from build123d import *

# Parameters (mm, degrees)
SKETCH1_R           = 6.35
SKETCH1_R_2         = 3.5814
EXTRUDE1_DEPTH      = 3.175
EXTRUDE1_DEPTH_BACK = 3.175
SKETCH4_W           = 1.1938
SKETCH4_H           = 7.9248
CHAMFER1_SIZE       = 0.254


with BuildPart() as part:
    # Sketch1 → Extrude1 (new, two sides)
    with BuildSketch(Plane(origin=(0, 0, 0), x_dir=(1, 0, 0), z_dir=(0, 1, 0))) as extrude1_sk:
        with Locations(Location((0, 0, 0), (0, 0, 270))):
            Circle(SKETCH1_R)
        with Locations(Location((0, 0, 0), (0, 0, 270))):
            Circle(SKETCH1_R_2, mode=Mode.SUBTRACT)
    extrude(amount=EXTRUDE1_DEPTH)
    extrude(extrude1_sk.sketch, amount=-EXTRUDE1_DEPTH_BACK)

    # Sketch4 → Revolve1 (revolve)
    with BuildSketch(Plane(origin=(0, 0, 0), x_dir=(1, 0, 0), z_dir=(0, 1, 0)), mode=Mode.PRIVATE) as revolve1_sk:
        with Locations((0.5969, -8.7376)):
            Rectangle(SKETCH4_W, SKETCH4_H)
    revolve(revolve1_sk.sketch.rotate(Axis((0, 0, 4.7752), (0, 0, 1)), 180), axis=Axis((0, 0, 4.7752), (0, 0, 1)))

    # Chamfer1
    chamfer1_edges = [part.edges().sort_by_distance(p)[0] for p in [
        (1.1938, 0, 12.7),
    ]]
    chamfer(chamfer1_edges, length=CHAMFER1_SIZE)


solid = part.part
Design review of the part built by this model. Coordinates are the model's own, in mm. Round coordinates to 2 decimals unless told otherwise and drop trailing zeros. Write each loop counter-clockwise with the first axis right and the second up, starting at its lowest first coordinate (ties: lowest second). Pieces come first, ordered by that corner, then holes. Notation, with made-up numbers: M -7.5,-0.5 L 47.5,-0.5 A30 ccw 47.5,32.5 Z; hole C 24,-33 d7. An arc over 180 degrees is marked long. One line per item, written item: value. Start each with the question number.
1. Draft analysis for pull direction Z (two halves, no side actions). For faces 1 (the face through (0, 0, 12.7)), 2 (the face through (0.259, 1.165, 9.298)), 3 (the face through (-3.18, -0.04, 1.65)), 4 (the face through (-3.86, 0.04, -5.04)), state which applies: pulls with the +Z half, pulls with the -Z half, needs draft (parallel to the pull), parting line crosses it, or undercut.
2. To check wall thickness, follow probe 1 along X at (y, z) = (1.25, 0); probe 2 along Z at (x, y) = (-2.25, -2.25); probe 3 along Z at (x, y) = (-1.25, 0.75). State the ranges of each line that lie inside material, in increasing order. Write a range as from..to.
3. Clearance check with flat-ended pins moving along their axes: P1, Ø1.5, axis at x = 1.5, y = -2, coming from the -Z side; P2, Ø1.5, axis at y = -0.5, z = 1, coming from the +X side; P3, Ø1, axis at x = -3, y = 1, coming from the -Z side. State where each tip first meets the part, or that it passes through.
4. Take a section at D-D on z = 7.5. State the section outline as (x, y) points.
5. Take a section at B-B on x = 0. State the section outline as (y, z) points (3 decimals), then the cut area to 3 significant figures.
6. Take a section at C-C on y = 0. State the section outline as (x, z) points, then the cut area to 3 significant figures.
7. Take a section at A-A on z = 0. State the section outline as (x, y) points (3 decimals).
Computed:
1. face 1: pulls with the +Z half
1. face 2: needs draft
1. face 3: undercut
1. face 4: parting line crosses it
2. probe 1: x = -6.35..-3.58, 3.58..6.35
2. probe 2: z = -5.94..-2.79, 2.79..5.94
2. probe 3: z = -6.23..-3.36, 3.36..6.23
3. P1: stops at z = -6.31
3. P2: stops at x = 6.35
3. P3: stops at z = -5.84
4. outline: C 0,0 d2.39
5. outline: M -3.175,-6.35 L 3.175,-6.35 L 3.175,-3.581 L -3.175,-3.581 Z; M -3.175,3.581 L 3.175,3.581 L 3.175,6.35 L 1.194,6.35 L 1.194,12.446 L 0.94,12.7 L -0.94,12.7 L -1.194,12.446 L -1.194,6.35 L -3.175,6.35 Z
5. area: 50.3 mm²
6. outline: M -1.19,6.24 A6.35 ccw long 1.19,6.24 L 1.19,12.45 L 0.94,12.7 L -0.94,12.7 L -1.19,12.45 Z; hole C 0,0 d7.16
6. area: 102 mm²
7. outline: M -6.35,-3.175 L -3.581,-3.175 L -3.581,3.175 L -6.35,3.175 Z; M 3.581,-3.175 L 6.35,-3.175 L 6.35,3.175 L 3.581,3.175 Z
